from build123d import *

# Parameters (mm, degrees)
CHAMFER_1_SIZE = 2


with BuildPart() as part:
    # 草图1 → 旋转1 (revolve)
    with BuildSketch(Plane.XY):
        Polygon((0, 0), (0, 10), (25, 10), (25, 8), (27, 8), (27, 17.5), (35, 17.5), (35, 13), (38, 13), (38, 15), (63, 15), (63, 0), align=None)
    revolve(axis=Axis((-82.844288888, 0, 0), (1, 0, 0)))

    # 倒角1
    chamfer_1_edges = [part.edges().sort_by_distance(p)[0] for p in [
        (0, -10, 0),
        (63, -15, 0),
    ]]
    chamfer(chamfer_1_edges, length=CHAMFER_1_SIZE)


solid = part.part
Work out the finished part from the listing and answer in its coordinate system (mm). A direction names the side the tool comes from. Round coordinates to 2 decimals unless told otherwise and drop trailing zeros. Write each loop counter-clockwise with the first axis right and the second up, starting at its lowest first coordinate (ties: lowest second). Pieces come first, ordered by that corner, then holes. Notation, with made-up numbers: (25.5, 38) -> (80.5, 38) arc R32 ccw to (80.5, 71) -> close; hole circle Ø4 at (85, -7.75). An arc over 180 degrees is marked (long way). Write each question's results on one line, items separated by ' | '.
Item 1: A cutting plane is placed at C-C, the plane x = 57. Determine the outline of the cut face in (y, z), plus the area to 3 significant figures.
Result set:
outline: circle Ø30 at (0, 0) | area: 707 mm^2
Item 2: A cutting plane is placed at A-A, the plane y = 0. Determine the outline of the cut face in (x, z), plus the area to 3 significant figures.
Result set:
outline: (0, -8) -> (2, -10) -> (25, -10) -> (25, -8) -> (27, -8) -> (27, -17.5) -> (35, -17.5) -> (35, -13) -> (38, -13) -> (38, -15) -> (61, -15) -> (63, -13) -> (63, 13) -> (61, 15) -> (38, 15) -> (38, 13) -> (35, 13) -> (35, 17.5) -> (27, 17.5) -> (27, 8) -> (25, 8) -> (25, 10) -> (2, 10) -> (0, 8) -> close | area: 1,630 mm^2
Item 3: Which of the six approach directions +Z, -Z, +X, -X, +Y, -Y give full straight-line access (tool end or side, diameter ignored) to faces 1 (the face through (27, -4, -8)), 2 (the face through (63, 0, 0)), 3 (the face through (49.661, -14.985, 0.66)), 4 (the face through (13.66, -2.17, -9.76))?
Result set:
face 1: none | face 2: +Z, -Z, +X, +Y, -Y | face 3: +X | face 4: -X
Item 4: Find the intervals of material crossed by line 1 along X through (y, z) = (-2, -11); line 2 along X through (y, z) = (5, -13); line 3 along X through (y, z) = (11.5, -12), in increasing order. Write a range as [from, to].
Result set:
line 1: [27, 63] | line 2: [27, 35], [38, 62.07] | line 3: [27, 35]
Item 5: The mould has two halves that part along X. Classify faces 5 (the face through (31.056, -13.887, -10.648)), 6 (the face through (0.13, -1.06, 8.06)), 7 (the face through (25, 0, 8.2)): +X half, -X half, draft (parallel to the pull), parting line (faces both ways), or undercut.
Result set:
face 5: draft | face 6: -X half | face 7: undercut
Item 6: Flat-ended cylindrical pins translate along their axes: P1, Ø3, axis at x = 9, z = 7.5, coming from the +Y side; P2, Ø10, axis at x = 42, z = 10, coming from the -Y side; P3, Ø5, axis at x = 6.5, y = 4.5, coming from the -Z side. Find the tip coordinate at first contact, or state that the pin passes through.
Result set:
P1: y = 8 | P2: y = -14.14 | P3: z = -9.8
Item 7: A cutting plane is placed at D-D, the plane x = 15. Determine the outline of the cut face in (y, z).
Result set:
outline: circle Ø20 at (0, 0)
